Can you work these out from the model? Positions are in its coordinate system, mm. Coordinates: 2 decimals unless noted, no trailing zeros. Loops run counter-clockwise (first coordinate to the right, second up) from the corner with the lowest first, then second, coordinate; pieces in that order, holes last. Notation, with made-up numbers: (30, 85.5) -> (71, 85.5) arc R9 ccw to (71, 91.5) -> close; hole circle Ø10 at (-20.75, 30.5). An arc over 180 degrees is marked (long way). Put each result on its own line as item: value. Start each with the question number.
Item 1: If we section it at A-A on y = 0: Please give me the cut outline in (x, z).
Item 2: If we section it at D-D on y = -28: Please give me the cut outline in (x, z).
Item 3: If we section it at C-C on x = 26.5: Please give me the cut outline in (y, z).
Item 4: Will these pins go through, and if not, where does the flat tip stop? P1, Ø1.8, axis at x = 47.92, y = -47.92, coming from the -Z side; P2, Ø0.8, axis at y = -43.5, z = 1, coming from the +X side.
Item 5: Please list where these lines run through material, in increasing order: L1, parallel to Y at x = 33, z = 0.45; L2, parallel to Y at x = 35, z = 0.85; L3, parallel to Y at x = 51.5, z = 1.55. Write a range as from..to.
Item 6: If we section it at B-B on z = 0.75: Please give me the cut outline in (x, y).
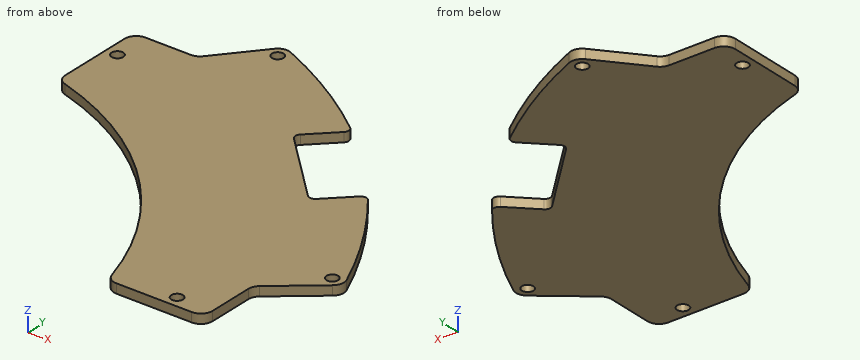
Autodesk Inventor part; units mm, degrees
ref_plane "YZ Plane" through (0, 0, 0) normal (1, 0, 0) x (0, 1, 0)
ref_plane "XZ Plane" through (0, 0, 0) normal (0, 1, 0) x (-1, 0, 0)
ref_plane "XY Plane" through (0, 0, 0) normal (0, 0, 1) x (1, 0, 0)
sketch "スケッチ1" plane through (0, 0, 0) normal (0, 0, 1) x (1, 0, 0)
  line L0 (54, -47.9205) -> (54, -40.1498)
  arc A0 (54.7258, -38.6082) -> (54, -40.1498) centre (56, -40.1498) ccw
  line L1 (54.7258, -38.6082) -> (62.3004, -32.3475)
  arc A1 (62.3004, -32.3475) -> (62.8611, -30.0103) centre (61.0262, -30.8059) ccw
  arc A2 (62.8611, -30.0103) -> (17.9102, 14.9406) centre (-16.5, -64.4205) ccw
  arc A3 (17.9102, 14.9406) -> (15.573, 14.3799) centre (17.1146, 13.1057) ccw
  line L2 (15.573, 14.3799) -> (9.3123, 6.8053)
  arc A4 (7.7707, 6.0795) -> (9.3123, 6.8053) centre (7.7707, 8.0795) ccw
  line L3 (7.7707, 6.0795) -> (0, 6.0795)
  arc A5 (0, 6.0795) -> (-2, 4.0795) centre (0, 4.0795) ccw
  line L4 (-2, 4.0795) -> (-2, -8.817)
  arc A6 (-2, -8.817) -> (-0.569, -10.7343) centre (0, -8.817) ccw
  arc A7 (37.1861, -48.4895) -> (-0.569, -10.7343) centre (-16.5, -64.4205) ccw
  arc A8 (37.1861, -48.4895) -> (39.1035, -49.9205) centre (39.1035, -47.9205) ccw
  line L5 (39.1035, -49.9205) -> (52, -49.9205)
  arc A9 (52, -49.9205) -> (54, -47.9205) centre (52, -47.9205) ccw
  circle A10 centre (47.9205, -47.9205) radius 1
  circle A11 centre (0, 0) radius 1
  circle A12 centre (17.1146, 13.1057) radius 1
  circle A13 centre (61.0262, -30.8059) radius 1
  point P0 (0, 0)
extrude "押し出し1" add sketch "スケッチ1" along normal blind 1.6
sketch "スケッチ2" plane through (0, 0, 1.6) normal (0, 0, 1) x (1, 0, 0)
  arc A0 (37.1861, -48.4895) -> (-0.569, -10.7343) centre (-16.5, -64.4205) ccw
  arc A1 (47.8768, -47.7509) -> (0, 0) centre (-16.5, -64.4205) ccw
sketch "スケッチ3" plane through (0, 0, 1.6) normal (0, 0, 1) x (1, 0, 0)
  circle A0 centre (42.5969, -6.8792) radius 0.375
  circle A1 centre (45.4254, -9.7076) radius 0.375
  circle A2 centre (38.3543, -2.6366) radius 0.375
  circle A3 centre (36.9401, -4.0508) radius 0.375
  circle A4 centre (44.0111, -11.1218) radius 0.375
  circle A5 centre (42.5969, -9.7076) radius 0.375
  circle A6 centre (41.1827, -8.2934) radius 0.375
  circle A7 centre (39.7685, -6.8792) radius 0.375
  circle A8 centre (38.3543, -5.465) radius 0.375
  circle A9 centre (44.0111, -8.2934) radius 0.375
  circle A10 centre (39.7685, -4.0508) radius 0.375
  circle A11 centre (41.1827, -5.465) radius 0.375
  line L0 (39.1035, -49.9205) -> (52, -49.9205)
  arc A12 (52, -49.9205) -> (54, -47.9205) centre (52, -47.9205) ccw
  line L1 (54, -47.9205) -> (54, -40.1498)
  arc A13 (54.7258, -38.6082) -> (54, -40.1498) centre (56, -40.1498) ccw
  line L2 (54.7258, -38.6082) -> (62.3004, -32.3475)
  arc A14 (62.3004, -32.3475) -> (62.8611, -30.0103) centre (61.0262, -30.8059) ccw
  arc A15 (62.8611, -30.0103) -> (17.9102, 14.9406) centre (-16.5, -64.4205) ccw
  arc A16 (17.9102, 14.9406) -> (15.573, 14.3799) centre (17.1146, 13.1057) ccw
  line L3 (15.573, 14.3799) -> (9.3123, 6.8053)
  arc A17 (7.7707, 6.0795) -> (9.3123, 6.8053) centre (7.7707, 8.0795) ccw
  line L4 (7.7707, 6.0795) -> (0, 6.0795)
  arc A18 (0, 6.0795) -> (-2, 4.0795) centre (0, 4.0795) ccw
  line L5 (-2, 4.0795) -> (-2, -8.817)
  arc A19 (-2, -8.817) -> (-0.569, -10.7343) centre (0, -8.817) ccw
  arc A20 (37.1861, -48.4895) -> (-0.569, -10.7343) centre (-16.5, -64.4205) ccw
  arc A21 (37.1861, -48.4895) -> (39.1035, -49.9205) centre (39.1035, -47.9205) ccw
  circle A22 centre (17.1146, 13.1057) radius 1
  circle A23 centre (61.0262, -30.8059) radius 1
  circle A24 centre (0, 0) radius 1
  circle A25 centre (47.9205, -47.9205) radius 1
  line L6 (44.6647, -3.2558) -> (23.098, -24.8225) construction
  line L7 (50.6967, -9.9517) -> (45.0399, -15.6085)
  line L8 (45.0399, -15.6085) -> (32.3119, -2.8806)
  line L9 (32.3119, -2.8806) -> (37.9688, 2.7762)
  arc A26 (62.8611, -30.0103) -> (17.9102, 14.9406) centre (-16.5, -64.4205) ccw
  point P0 (0, 0)
  dimension "d2" = 18
  dimension "d3" = 8
extrude "押し出し2" cut sketch "スケッチ3" against normal up to surface (1.6 mm away) contours A0 | A1 | A2 | A3 | A4 | A5 | A6 | A7 | A8 | A9 | A10 | A11 | L7 L8 L9 A15
fillet "フィレット1" radius 1 4 edges at (50.6967, -9.9517, 0.8) (45.0399, -15.6085, 0.8) (32.3119, -2.8806, 0.8) (37.9688, 2.7762, 0.8)
properties part number "MotorDriver_PCB"
Solutions:
1. outline: (-2, 0) -> (-1, 0) -> (-1, 1.6) -> (-2, 1.6) -> close; (1, 0) -> (35.19, 0) -> (35.19, 1.6) -> (1, 1.6) -> close
2. outline: (26.04, 0) -> (61.96, 0) -> (61.96, 1.6) -> (26.04, 1.6) -> close
3. outline: (-28.55, 0) -> (10.63, 0) -> (10.63, 1.6) -> (-28.55, 1.6) -> close
4. P1: through
4. P2: x = 54
5. L1: -38.23..-3.57, -2.19..6.52
5. L2: -42.43..-5.57, -0.19..5.08
5. L3: -49.92..-10.96
6. outline: (-2, -8.82) arc R2 ccw to (-0.57, -10.73) arc R56 cw to (37.19, -48.49) arc R2 ccw to (39.1, -49.92) -> (52, -49.92) arc R2 ccw to (54, -47.92) -> (54, -40.15) arc R2 cw to (54.73, -38.61) -> (62.3, -32.35) arc R2 ccw to (62.86, -30.01) arc R86.5 ccw to (51.4, -10.83) arc R1 ccw to (49.91, -10.74) -> (45.75, -14.9) arc R1 cw to (44.33, -14.9) -> (33.02, -3.59) arc R1 cw to (33.02, -2.17) -> (37.18, 1.99) arc R1 ccw to (37.09, 3.48) arc R86.5 ccw to (17.91, 14.94) arc R2 ccw to (15.57, 14.38) -> (9.31, 6.81) arc R2 cw to (7.77, 6.08) -> (0, 6.08) arc R2 ccw to (-2, 4.08) -> close; hole circle Ø2 at (0, 0); hole circle Ø2 at (17.11, 13.11); hole circle Ø2 at (47.92, -47.92); hole circle Ø2 at (61.03, -30.81)
